from build123d import *

# Parameters (mm, degrees)
EXTRUDE_1_DEPTH     = 200
SKETCH_2_R          = 2.25
CUT_EXTRUDE_1_DEPTH = 16


with BuildPart() as part:
    # Эскиз1 → Бобышка-Вытянуть1 (new body)
    with BuildSketch(Plane(origin=(0, 0, 0), x_dir=(0, 0, -1), z_dir=(1, 0, 0))):
        Polygon((0, 0), (0, 15), (1.5, 15), (1.5, 1.5), (15, 1.5), (15, 0), align=None)
    extrude(amount=EXTRUDE_1_DEPTH)

    # Эскиз2 → Вырез-Вытянуть1 (cut, through all)
    with BuildSketch(Plane.XZ):
        with Locations((7.5, -7.5)):
            Circle(SKETCH_2_R)
        with Locations((192.5, -7.5)):
            Circle(SKETCH_2_R)
    extrude(amount=-CUT_EXTRUDE_1_DEPTH, mode=Mode.SUBTRACT)


solid = part.part
Read the model definition and answer for the solid it produces. Units are mm, in the model's axes. A direction names the side the tool comes from. Coordinates: 2 decimals unless noted, no trailing zeros. Loops run counter-clockwise (first coordinate to the right, second up) from the corner with the lowest first, then second, coordinate; pieces in that order, holes last.
Q1. The part is cut by section B-B on x = 7.5. Write down the section's boundary in (y, z), and give its area (3 significant figures).
Q2. The part is cut by section A-A on z = -7.5. Write down the section's boundary in (x, y), and give its area (4 significant figures).
Q3. The mould has two halves that part along X. Classify faces 1 (the face through (99, 1.5, -8)), 2 (the face through (194.646, 0.74, -6.824)), 3 (the face through (200, 1, -4)): +X half, -X half, draft (parallel to the pull), parting line (faces both ways), or undercut.
Q4. Consider probe 1 along Z at (x, y) = (7.5, 1.15); probe 2 along Y at (x, z) = (189, -7); probe 3 along Z at (x, y) = (191, 7.5). Determine where each line is inside the solid, lowest interval first.
Q5. The part is cut by section D-D on y = 10.75. Write down the section's boundary in (x, z).
Q6. Each of these flat-tipped pins is pushed along its axis until it touches: pin 1 Ø5 at (x, z) = (115, -6.5) entering from +Y; pin 2 Ø2 at (x, y) = (46.5, 7.5) entering from -Z. Where does it stop, or does it pass through?
Q7. The part is cut by section C-C on x = 101. Write down the section's boundary in (y, z).
Q8. Which of the six approach directions +Z, -Z, +X, -X, +Y, -Y give full straight-line access (tool end or side, diameter ignored) to faces 4 (the face through (99, 0, -8)), 5 (the face through (99, 8, -1.5))?
Results below:
1. outline: (0, -15) - (1.5, -15) - (1.5, -9.75) - (0, -9.75) - close; (0, -5.25) - (1.5, -5.25) - (1.5, -1.5) - (15, -1.5) - (15, 0) - (0, 0) - close
1. area: 36.0 mm2
2. outline: (0, 0) - (5.25, 0) - (5.25, 1.5) - (0, 1.5) - close; (9.75, 0) - (190.25, 0) - (190.25, 1.5) - (9.75, 1.5) - close; (194.75, 0) - (200, 0) - (200, 1.5) - (194.75, 1.5) - close
2. area: 286.5 mm2
3. face 1: draft
3. face 2: undercut
3. face 3: +X half
4. probe 1: z = -15 to -9.75, -5.25 to 0
4. probe 2: y = 0 to 1.5
4. probe 3: z = -1.5 to 0
5. outline: (0, -1.5) - (200, -1.5) - (200, 0) - (0, 0) - close
6. pin 1: stops at y = 1.5
6. pin 2: stops at z = -1.5
7. outline: (0, -15) - (1.5, -15) - (1.5, -1.5) - (15, -1.5) - (15, 0) - (0, 0) - close
8. face 4: +Z, -Z, +X, -X, -Y
8. face 5: -Z, +X, -X, +Y
